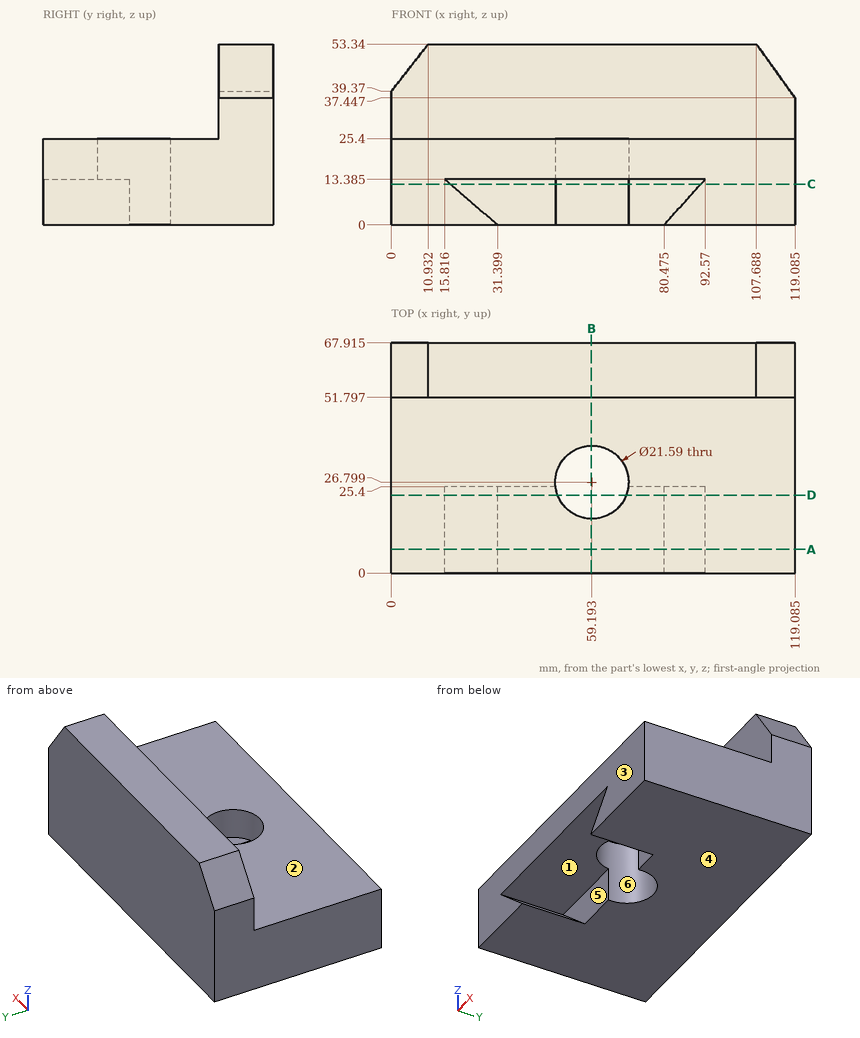
Input: dimensioned drawing with shaded views. Units: mm. Origin: part minimum x, y, z. A direction names the side the tool comes from. Round coordinates to 2 decimals unless told otherwise and drop trailing zeros. Loops run counter-clockwise (first coordinate to the right, second up) from the corner with the lowest first, then second, coordinate; pieces in that order, holes last. Notation, with made-up numbers: M -6,61 L 35,61 A24 ccw 35,79 Z; hole C -29.5,-32 d7. An arc over 180 degrees is marked long. One line per question, with ' | ' between items.
(1) Pull-direction query (Y, two-part tool) for the marked faces 4, 5 and 6; classes: +Y half, -Y half, draft (parallel to the pull), parting line (faces both ways), or undercut.
Check result:
face 4: draft | face 5: -Y half | face 6: undercut
(2) Contact query for flat-ended pins moving along their axis: P1, Ø1.5, axis at x = 19.5, y = 33.5, coming from the +Z side; P2, Ø8.5, axis at x = 81.5, z = 34, coming from the -Y side; P3, Ø13, axis at x = 59.19, y = 26.8, coming from the +Z side. Output: stop coordinate, or through.
Check result:
P1: stops at z = 25.4 | P2: stops at y = 51.8 | P3: passes through
(3) Cut plane C-C on z = 12. Return the cut outline in (x, y) (1 decimal).
Check result:
outline: M 0,0 L 17.4,0 L 17.4,25.4 L 48.5,25.4 A10.8 cw long 69.9,25.4 L 91.3,25.4 L 91.3,0 L 119.1,0 L 119.1,67.9 L 0,67.9 Z
(4) Material intervals for line 1 along X through (y, z) = (26.5, 23) (1 decimal); line 2 along Y through (x, z) = (10, 44.5) (1 decimal); line 3 along Z through (x, y) = (7, 31), sorted ascending. Write a range as from..to.
Check result:
line 1: x = 0..48.4, 70..119.1 | line 2: y = 51.8..67.9 | line 3: z = 0..25.4
(5) Cut plane B-B on x = 59. Return the cut outline in (y, z) (1 decimal).
Check result:
outline: M 0,13.4 L 16,13.4 L 16,25.4 L 0,25.4 Z; M 37.6,0 L 67.9,0 L 67.9,53.3 L 51.8,53.3 L 51.8,25.4 L 37.6,25.4 Z
(6) Access query for the marked faces 1, 2 and 3. Directions: +Z, -Z, +X, -X, +Y, -Y. A direction counts if a zero-diameter tool reaches every point of the face in a straight line with its end or side. Return the directions, or none.
Check result:
face 1: -Y | face 2: +Z, +X, -X, -Y | face 3: +Z, -Z, +X, -X, -Y
(7) Cut plane A-A on y = 7. Return the cut outline in (x, z) (1 decimal).
Check result:
outline: M 0,0 L 31.4,0 L 15.8,13.4 L 92.6,13.4 L 80.5,0 L 119.1,0 L 119.1,25.4 L 0,25.4 Z
(8) Cut plane D-D on y = 23. Return the cut outline in (x, z) (1 decimal), plus the area to 3 significant figures.
Check result:
outline: M 0,0 L 31.4,0 L 15.8,13.4 L 49.1,13.4 L 49.1,25.4 L 0,25.4 Z; M 69.3,13.4 L 92.6,13.4 L 80.5,0 L 119.1,0 L 119.1,25.4 L 69.3,25.4 Z | area: 1,940 mm2
